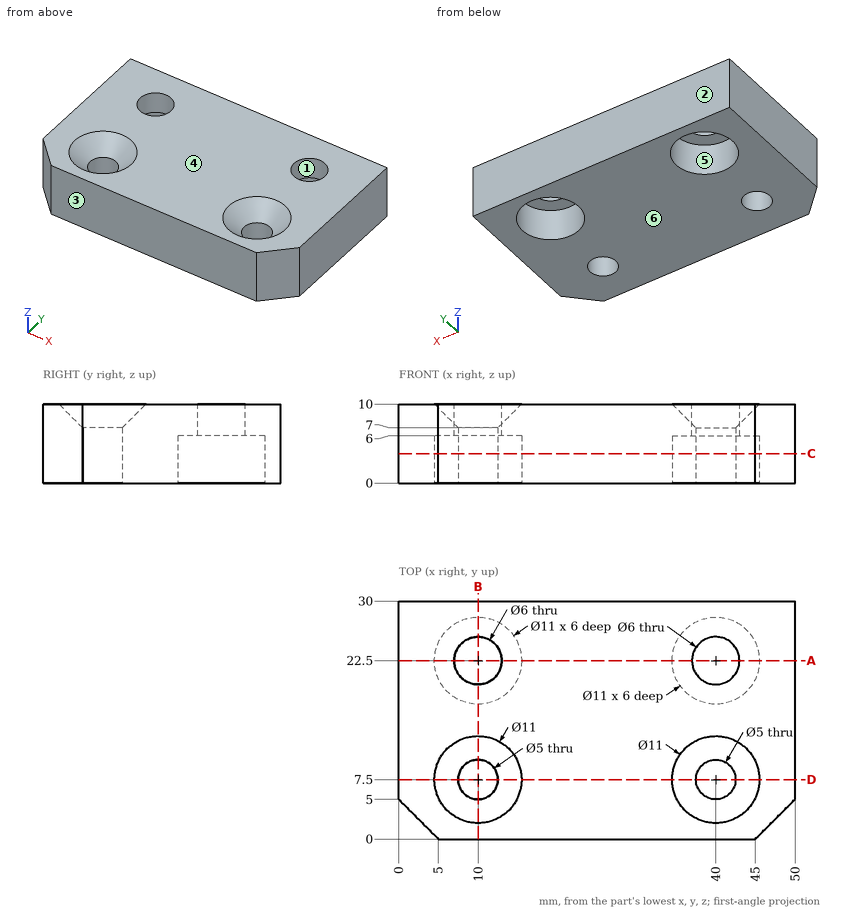
Part print with two shaded views. Sizes in mm from the minimum x, y, z corner. A direction names the side the tool comes from. Give positions to 0.01 mm unless a question says otherwise; leave off trailing zeros. Order: outer loops, then holes, each group sorted by start corner. A loop starts at its lowest first (then second) coordinate and runs counter-clockwise, first axis right, second up. Notation, with made-up numbers: M 58.5,4 L 71.5,4 A14 cw 71.5,18 Z; hole C -40,67.25 d1. An arc over 180 degrees is marked long. Put each result on its own line as item: value.
Item 1: Wall check: probe 1 along Y at (x, z) = (40, 2.25); probe 2 along X at (y, z) = (7.5, 4.25); probe 3 along Y at (x, z) = (10, 6.95). Give the ranges that are in metal, low to high.
Results are:
probe 1: 0 to 5, 10 to 17, 28 to 30
probe 2: 0 to 7.5, 12.5 to 37.5, 42.5 to 50
probe 3: 0 to 5, 10 to 19.5, 25.5 to 30
Item 2: Drop flat-ended pins along their axis: pin 1 Ø5.5 at (x, y) = (8.5, 20.5) entering from -Z; pin 2 Ø6.5 at (x, y) = (40, 7.5) entering from +Z. Give the stop position or say it passes through.
Results are:
pin 1: z = 6
pin 2: z = 7.75
Item 3: Cut at A-A on y = 22.5. Write the cut outline in (x, z).
Results are:
outline: M 0,0 L 4.5,0 L 4.5,6 L 7,6 L 7,10 L 0,10 Z; M 13,6 L 15.5,6 L 15.5,0 L 34.5,0 L 34.5,6 L 37,6 L 37,10 L 13,10 Z; M 43,6 L 45.5,6 L 45.5,0 L 50,0 L 50,10 L 43,10 Z
Item 4: Cut at C-C on z = 3.75. Write the cut outline in (x, y), then the cut area to 3 significant figures.
Results are:
outline: M 0,5 L 5,0 L 45,0 L 50,5 L 50,30 L 0,30 Z; hole C 10,22.5 d11; hole C 10,7.5 d5; hole C 40,22.5 d11; hole C 40,7.5 d5
area: 1,250 mm2
Item 5: Cut at D-D on y = 7.5. Write the cut outline in (x, z), then the cut area to 3 significant figures.
Results are:
outline: M 0,0 L 7.5,0 L 7.5,7 L 4.5,10 L 0,10 Z; M 12.5,0 L 37.5,0 L 37.5,7 L 34.5,10 L 15.5,10 L 12.5,7 Z; M 42.5,0 L 50,0 L 50,10 L 45.5,10 L 42.5,7 Z
area: 382 mm2
Item 6: Cut at B-B on x = 10. Write the cut outline in (y, z).
Results are:
outline: M 0,0 L 5,0 L 5,7 L 2,10 L 0,10 Z; M 10,0 L 17,0 L 17,6 L 19.5,6 L 19.5,10 L 13,10 L 10,7 Z; M 25.5,6 L 28,6 L 28,0 L 30,0 L 30,10 L 25.5,10 Z
Item 7: Which spindle directions (+Z, -Z, +X, -X, +Y, -Y) get a long thin tool onto all of the face, cutting with end or side? Do the marked faces 5 and 6. Say none if no direction does.
Results are:
face 5: -Z
face 6: -Z, +X, -X, +Y, -Y
Item 8: Pull direction Y, two halves, no side cores. Call the marked faces 1, 2, 3 and 4: +Y half, -Y half, draft (parallel to the pull), parting line (faces both ways), or undercut.
Results are:
face 1: undercut
face 2: +Y half
face 3: -Y half
face 4: draft
